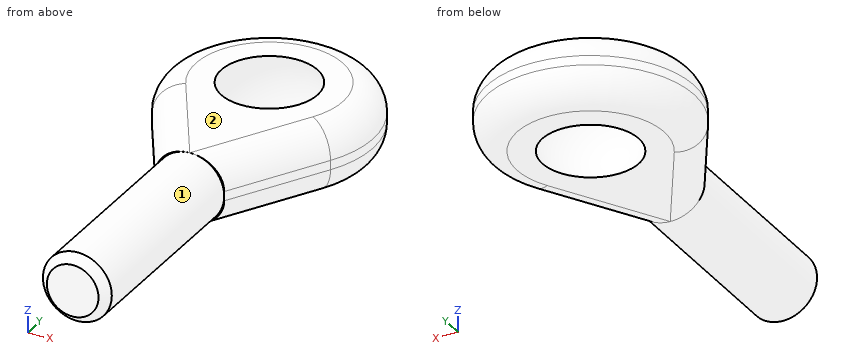
from build123d import *

# Parameters (mm, degrees)
SKETCH1_R           = 4
BOSS_EXTRUDE1_DEPTH = 12.5
BOSS_EXTRUDE6_DEPTH = 4
CHAMFER1_SIZE       = 1
FILLET6_R           = 3.4584


with BuildPart() as part:
    # Sketch1 → Boss-Extrude1 (new body, symmetric)
    with BuildSketch(Plane(origin=(0, 0, 0), x_dir=(1, 0, 0), z_dir=(0, 1, 0))):
        Circle(SKETCH1_R)
    extrude(amount=BOSS_EXTRUDE1_DEPTH, both=True)

    # Sketch10 → Boss-Extrude6 (add, symmetric)
    with BuildSketch(Plane.XY):
        with BuildLine():
            Line((-10.37531088, 23.470661383), (-4, 12.5))
            Line((-4, 12.5), (4, 12.5))
            Line((4, 12.5), (10.37531088, 23.470661383))
            ThreePointArc((10.37531088, 23.470661383), (0, 41.5), (-10.37531088, 23.470661383))
        make_face()
    extrude(amount=BOSS_EXTRUDE6_DEPTH, both=True)

    # Chamfer1
    chamfer1_edges = [part.edges().sort_by_distance(p)[0] for p in [
        (-4, -12.5, 0),
    ]]
    chamfer(chamfer1_edges, length=CHAMFER1_SIZE)

    # Sketch11 → Cut-Revolve1 (revolve, cut)
    with BuildSketch(Plane(origin=(0, 0, 0), x_dir=(0, 0, -1), z_dir=(1, 0, 0))):
        with BuildLine():
            Line((-4.5, 29.5), (4.5, 29.5))
            Line((4.5, 29.5), (4.5, 34.7))
            ThreePointArc((4.5, 34.7), (0, 36.376772499), (-4.5, 34.7))
            Line((-4.5, 34.7), (-4.5, 29.5))
        make_face()
    revolve(axis=Axis((0, 29.5, 4.5), (0, 0, -1)), mode=Mode.SUBTRACT)

    # Fillet6
    fillet6_edges = [part.edges().sort_by_distance(p)[0] for p in [
        (-7.18765544, 17.985330692, 4),
        (0, 41.5, 4),
        (7.18765544, 17.985330692, 4),
        (7.18765544, 17.985330692, -4),
        (0, 41.5, -4),
        (-7.18765544, 17.985330692, -4),
    ]]
    fillet(fillet6_edges, radius=FILLET6_R)


solid = part.part
Geometry check sheet. Reference: the model listing, model coordinates, mm. Face numbers are marked on the shaded views. A direction names the side the tool comes from. Give positions to 0.01 mm unless a question says otherwise; leave off trailing zeros. Write each loop counter-clockwise with the first axis right and the second up, starting at its lowest first coordinate (ties: lowest second). Pieces come first, ordered by that corner, then holes.
1) Set-up check for the marked faces 1 and 2: record each of +Z, -Z, +X, -X, +Y, -Y from which the full face is reachable in a straight line by a thin tool's end or side.
Values follow:
face 1: -Y
face 2: +Z, +X, -X, +Y, -Y
2) Cross-section at A-A (y = -6). Record the boundary of the cut face in (x, z).
Values follow:
outline: circle Ø8 at (0, 0)
3) Thickness scan on line 1 (X direction, y = 33.5, z = -1.25); line 2 (Y direction, x = 3, z = 0.5); line 3 (Y direction, x = 1, z = 3). Record the ranges inside material, lowest first.
Values follow:
line 1: x = -11.24 to -5.45, 5.45 to 11.24
line 2: y = -12.46 to 23.33, 35.67 to 41.12
line 3: y = -12.34 to 23.39, 35.61 to 40.43
